Read the model definition and answer for the solid it produces. Units are mm, in the model's axes. A direction names the side the tool comes from. Give positions to 0.01 mm unless a question says otherwise; leave off trailing zeros. Order: outer loops, then holes, each group sorted by start corner. A loop starts at its lowest first (then second) coordinate and runs counter-clockwise, first axis right, second up. Notation, with made-up numbers: (16, 2.5) -> (70, 2.5) arc R20 ccw to (70, 22.5) -> close; hole circle Ø2 at (-26.75, -9). An arc over 180 degrees is marked (long way). Use one line per item in the form item = value.
```python
from build123d import *

# Parameters (mm, degrees)
F1_DEPTH = 3


with BuildPart() as f1:
    # F0 (on Top) → F1 (new body)
    with BuildSketch(Plane.XY):
        Polygon((10, 17), (10, 20), (2.5, 20), (2.5, 19), (2.5, 18), (0, 16), (-2.5, 18), (-2.5, 19), (-2.5, 19.7), (-2.5, 20), (-10, 20), (-10, 17), (-27, 17), (-27, 7.5), (-30, 7.5), (-30, -7.5), (-27, -7.5), (-27, -17), (-10, -17), (-10, -20), (10, -20), (10, -17), (27, -17), (27, -7.5), (30, -7.5), (30, 7.5), (27, 7.5), (27, 17), align=None)
        Polygon((0, 16), (2.5, 18), (0, 18), align=None)
        Polygon((0, 16), (0, 18), (-2.5, 18), align=None)
        Polygon((-2.5, 18), (0, 18), (0, 20), (-1, 20), (-1, 19), (-2.5, 19), align=None)
        Polygon((2.5, 18), (2.5, 19), (1, 19), (1, 20), (0, 20), (0, 18), align=None)
        Polygon((0, 20), (1, 20), (1, 21), (2.5, 21), (2.5, 22), (-2.5, 22), (-2.5, 21), (-1, 21), (-1, 20), align=None)
    extrude(amount=F1_DEPTH)


solid = f1.part
```
Item 1: The part is cut by section C-C on y = -16. Give the vertices of the cut face in (x, z), and give its area (3 significant figures).
Checks:
outline = (-27, 0) -> (27, 0) -> (27, 3) -> (-27, 3) -> close
area = 162 mm²
Item 2: Straight lines are drawn through the part: L1, parallel to Y at x = -2, z = 0.7; L2, parallel to X at y = 13.5, z = 0.15; L3, parallel to X at y = 17.5, z = 1.8. For each, find the intervals that lie inside material, in ascending order. Write a range as from..to.
Checks:
L1 = -20..19, 21..22
L2 = -27..27
L3 = -10..10
Item 3: The part is cut by section B-B on x = 19. Give the vertices of the cut face in (y, z).
Checks:
outline = (-17, 0) -> (17, 0) -> (17, 3) -> (-17, 3) -> close
Item 4: Determine the mould class of faces 1 (the flat face through (-1, 20, 1)), 2 (the flat face through (6, 20, 1)), 3 (the flat face through (18, -17, 1)), 4 (the flat face through (-2, 19, 1)) for opening direction Y: +Y half, -Y half, draft (parallel to the pull), parting line (faces both ways), or undercut.
Checks:
face_1 = undercut
face_2 = +Y half
face_3 = -Y half
face_4 = undercut
Item 5: Which of the six approach directions +Z, -Z, +X, -X, +Y, -Y give full straight-line access (tool end or side, diameter ignored) to faces 5 (the flat face through (27, 12, 1)), 6 (the flat face through (27, -12, 1)), 7 (the flat face through (-10, -18, 1)), 8 (the flat face through (-27, 12, 1))?
Checks:
face_5 = +Z, -Z, +X, +Y
face_6 = +Z, -Z, +X, -Y
face_7 = +Z, -Z, -X, -Y
face_8 = +Z, -Z, -X, +Y
Item 6: Given pin 1 Ø0.8 at (y, z) = (21.5, 1.5) entering from +X; pin 2 Ø1.6 at (y, z) = (20.5, 1.5) entering from +X; pin 3 Ø1.5 at (x, z) = (-6, 1) entering from +Y, each flat-ended and moving along its own axis, determine where each tip first touches the part or whether it passes through.
Checks:
pin_1 = 2.5
pin_2 = 10
pin_3 = 20
